Geometry check sheet. Reference: the model listing, model coordinates, mm. A direction names the side the tool comes from. Round coordinates to 2 decimals unless told otherwise and drop trailing zeros. Loops run counter-clockwise (first coordinate to the right, second up) from the corner with the lowest first, then second, coordinate; pieces in that order, holes last. Notation, with made-up numbers: M 80.5,78 L 126.5,78 A32 cw 126.5,104 Z; hole C 37.5,-27.5 d6. An arc over 180 degrees is marked long. Write item = value, one per line.
from build123d import *

# Parameters (mm, degrees)
SKETCH3_R           = 12.7
SKETCH3_R_2         = 0.975
BOSS_EXTRUDE2_DEPTH = 1.5875


with BuildPart() as part:
    # Sketch3 → Boss-Extrude2 (new body)
    with BuildSketch(Plane.XY):
        Circle(SKETCH3_R)
        with BuildLine():
            ThreePointArc((6.269554118, 8.885849209), (0, 10.875), (-6.269554118, 8.885849209))
            Line((-6.269554118, 8.885849209), (-5.055813485, 7.672108576))
            ThreePointArc((-5.055813485, 7.672108576), (-5.055813485, 5.055813485), (-7.672108576, 5.055813485))
            Line((-7.672108576, 5.055813485), (-8.885849209, 6.269554118))
            ThreePointArc((-8.885849209, 6.269554118), (-10.875, 0), (-8.885849209, -6.269554118))
            Line((-8.885849209, -6.269554118), (-7.672108576, -5.055813485))
            ThreePointArc((-7.672108576, -5.055813485), (-5.055813485, -5.055813485), (-5.055813485, -7.672108576))
            Line((-5.055813485, -7.672108576), (-6.269554118, -8.885849209))
            ThreePointArc((-6.269554118, -8.885849209), (0, -10.875), (6.269554118, -8.885849209))
            Line((6.269554118, -8.885849209), (5.055813485, -7.672108576))
            ThreePointArc((5.055813485, -7.672108576), (5.055813485, -5.055813485), (7.672108576, -5.055813485))
            Line((7.672108576, -5.055813485), (8.885849209, -6.269554118))
            ThreePointArc((8.885849209, -6.269554118), (10.875, 0), (8.885849209, 6.269554118))
            Line((8.885849209, 6.269554118), (7.672108576, 5.055813485))
            ThreePointArc((7.672108576, 5.055813485), (5.055813485, 5.055813485), (5.055813485, 7.672108576))
            Line((5.055813485, 7.672108576), (6.269554118, 8.885849209))
        make_face(mode=Mode.SUBTRACT)
        with BuildLine():
            Line((5.055813485, 7.672108576), (6.269554118, 8.885849209))
            ThreePointArc((6.269554118, 8.885849209), (0, 10.875), (-6.269554118, 8.885849209))
            Line((-6.269554118, 8.885849209), (-5.055813485, 7.672108576))
            ThreePointArc((-5.055813485, 7.672108576), (-5.055813485, 5.055813485), (-7.672108576, 5.055813485))
            Line((-7.672108576, 5.055813485), (-8.885849209, 6.269554118))
            ThreePointArc((-8.885849209, 6.269554118), (-10.875, 0), (-8.885849209, -6.269554118))
            Line((-8.885849209, -6.269554118), (-7.672108576, -5.055813485))
            ThreePointArc((-7.672108576, -5.055813485), (-5.055813485, -5.055813485), (-5.055813485, -7.672108576))
            Line((-5.055813485, -7.672108576), (-6.269554118, -8.885849209))
            ThreePointArc((-6.269554118, -8.885849209), (0, -10.875), (6.269554118, -8.885849209))
            Line((6.269554118, -8.885849209), (5.055813485, -7.672108576))
            ThreePointArc((5.055813485, -7.672108576), (5.055813485, -5.055813485), (7.672108576, -5.055813485))
            Line((7.672108576, -5.055813485), (8.885849209, -6.269554118))
            ThreePointArc((8.885849209, -6.269554118), (10.875, 0), (8.885849209, 6.269554118))
            Line((8.885849209, 6.269554118), (7.672108576, 5.055813485))
            ThreePointArc((7.672108576, 5.055813485), (5.055813485, 5.055813485), (5.055813485, 7.672108576))
        make_face()
        with Locations((0, 9.000000134)):
            Circle(SKETCH3_R_2, mode=Mode.SUBTRACT)
        with Locations((9.000000134, 0)):
            Circle(SKETCH3_R_2, mode=Mode.SUBTRACT)
        with Locations((0, -9.000000134)):
            Circle(SKETCH3_R_2, mode=Mode.SUBTRACT)
        with Locations((-9.000000134, 0)):
            Circle(SKETCH3_R_2, mode=Mode.SUBTRACT)
        with BuildLine():
            ThreePointArc((6.850845531, 1.663855614), (6.830865544, 1.714608205), (6.79791666, 1.758075393))
            Line((6.79791666, 1.758075393), (1.758075393, 6.79791666))
            ThreePointArc((1.758075393, 6.79791666), (1.714608205, 6.830865544), (1.663855614, 6.850845531))
            ThreePointArc((1.663855614, 6.850845531), (-4.985102807, 4.985102807), (-6.850845531, -1.663855614))
            ThreePointArc((-6.850845531, -1.663855614), (-6.830865544, -1.714608205), (-6.79791666, -1.758075393))
            Line((-6.79791666, -1.758075393), (-1.758075393, -6.79791666))
            ThreePointArc((-1.758075393, -6.79791666), (-1.714608205, -6.830865544), (-1.663855614, -6.850845531))
            ThreePointArc((-1.663855614, -6.850845531), (4.985102807, -4.985102807), (6.850845531, 1.663855614))
        make_face(mode=Mode.SUBTRACT)
    extrude(amount=BOSS_EXTRUDE2_DEPTH)


solid = part.part
(1) Release check for a two-part mould opening along Y. For faces 1 (the flat face through (5.5, -5.5, 1.588)), 2 (the cylindrical face through (-2.75, -12.4, 0.78)), 3 (the cylindrical face through (-4.91, 5.06, 0.78)), 4 (the cylindrical face through (-8.07, 0.29, 0.78)) record: released by +Y, released by -Y, zero draft, split by the parting line, or undercut.
Result set:
face_1 = zero draft
face_2 = split by the parting line
face_3 = undercut
face_4 = undercut
(2) Material ranges on line 1 along Y through (x, z) = (0, 1.3) (3 decimals); line 2 along Y through (x, z) = (-0.25, 1.55); line 3 along X through (y, z) = (-0.5, 0.3), recorded low to high. Write a range as from..to.
Result set:
line_1 = -12.7..-9.975, -8.025..-7.05, 7.05..8.025, 9.975..12.7
line_2 = -12.7..-9.94, -8.06..-7.05, 7.05..8.06, 9.94..12.7
line_3 = -12.69..-9.84, -8.16..-7.03, 7.03..8.16, 9.84..12.69
(3) Tool access check on faces 5 (the flat face through (-4.313, -4.243, 0.783)), 6 (the flat face through (5.5, -5.5, 0)). Record the directions out of +Z, -Z, +X, -X, +Y, -Y that give a thin tool (end or side, any length) a straight path to the whole face; none if there is none.
Result set:
face_5 = +Z, -Z
face_6 = -Z, +X, -X, +Y, -Y
(4) Sectioned sample at A-A on y = 0. State how many separate pieces and enclosed holes the cut face has, then the cut area to 3 significant figures.
Result set:
separate_pieces = 4
enclosed_holes = 0
area = 11.7 mm2
(5) Depth check by flat-ended pin: pin 1 Ø1.8 at (x, y) = (9, 0) entering from +Z. Enter the tip coordinate at first touch or a pass-through.
Result set:
pin_1 = through
(6) Sectioned sample at D-D on x = 9. Record the cut outline in (y, z) (1 decimal).
Result set:
outline = M -9,0 L -1,0 L -1,1.6 L -9,1.6 Z; M 1,0 L 9,0 L 9,1.6 L 1,1.6 Z
